```python
from build123d import *

# Parameters (mm, degrees)
SKETCH_1_W               = 120
SKETCH_1_H               = 80
EXTRUDE_1_DEPTH          = 5
SKETCH_3_R               = 4
CUT_EXTRUDE_2_DEPTH      = 10
SKETCH_5_R               = 15
CUT_EXTRUDE_3_DEPTH      = 10
F_4_0MM_1_D              = 4
FILLET_1_R               = 10
SKETCH_13_R              = 6.969385005
EXTRUDE_5_DEPTH          = 5
SKETCH_14_W              = 5
SKETCH_14_H              = 75
EXTRUDE_6_DEPTH          = 80
SKETCH_15_W              = 20
SKETCH_15_H              = 5
EXTRUDE_7_DEPTH          = 80
EXTRUDE_8_DEPTH          = 5
FILLET_2_R               = 1
F_3_0MM_1_D              = 3
F_3_0MM_1_DEPTH          = 7.5
F_3_0MM_1_TIP            = 0.901290929
SKETCH_21_R              = 2.5
CUT_EXTRUDE_7_DEPTH      = 10
PATTERN_CIRCULAR_1_COUNT = 4


with BuildPart() as part:
    # 草图1 → 凸台-拉伸1 (new body)
    with BuildSketch(Plane.XY):
        Rectangle(SKETCH_1_W, SKETCH_1_H)
    extrude(amount=EXTRUDE_1_DEPTH)

    # 草图3 → 切除-拉伸2 (cut)
    with BuildSketch(Plane.XY.offset(5)):
        with Locations((-45, 0)):
            Circle(SKETCH_3_R)
    extrude(amount=-CUT_EXTRUDE_2_DEPTH, mode=Mode.SUBTRACT)

    # 草图5 → 切除-拉伸3 (cut)
    with BuildSketch(Plane.XY.offset(5)):
        with Locations((35, 0)):
            Circle(SKETCH_5_R)
    extrude(amount=-CUT_EXTRUDE_3_DEPTH, mode=Mode.SUBTRACT)

    # Ø4.0mm 暗销孔1 (through all)
    with Locations(Plane(origin=(0, 0, 0), x_dir=(-1, 0, 0), z_dir=(0, 0, -1))):
        with Locations((-8.5, -22.25), (-8.5, 22.25), (-33.5, 22.25), (-33.5, -22.25)):
            Hole(F_4_0MM_1_D / 2)

    # 圆角1
    fillet_1_edges = [part.edges().sort_by_distance(p)[0] for p in [
        (-60, 40, 2.5),
        (-60, -40, 2.5),
    ]]
    fillet(fillet_1_edges, radius=FILLET_1_R)

    # 草图13 → 凸台-拉伸5 (add)
    with BuildSketch(Plane.XY.offset(5)):
        with Locations((-45, 0)):
            Circle(SKETCH_13_R)
    extrude(amount=-EXTRUDE_5_DEPTH)

    # 草图14 → 凸台-拉伸6 (add)
    with BuildSketch(Plane.XZ.offset(40)):
        with Locations((57.5, -37.5)):
            Rectangle(SKETCH_14_W, SKETCH_14_H)
    extrude(amount=-EXTRUDE_6_DEPTH)

    # 草图15 → 凸台-拉伸7 (add)
    with BuildSketch(Plane.XZ.offset(40)):
        with Locations((45, -72.5)):
            Rectangle(SKETCH_15_W, SKETCH_15_H)
    extrude(amount=-EXTRUDE_7_DEPTH)

    # 草图16 → 凸台-拉伸8 (add)
    with BuildSketch(Plane.XZ.offset(40)):
        Polygon((20, 5), (20, 0), (35, -55), (35, -75), (60, -75), (60, 5), align=None)
    extrude_8 = extrude(amount=-EXTRUDE_8_DEPTH)

    # 镜向1: 凸台-拉伸8 across plane
    add(extrude_8.mirror(Plane.ZX))

    # 圆角2
    fillet_2_edges = [part.edges().sort_by_distance(p)[0] for p in [
        (27.5, -40, -27.5),
        (-15, 40, 0),
        (60, 0, 5),
        (27.5, 40, -27.5),
        (5, 40, 5),
        (-15, -40, 0),
        (5, -40, 5),
        (-60, 0, 0),
        (-57.071067812, 37.071067812, 0),
        (-57.071067812, -37.071067812, 0),
        (-60, 0, 5),
        (-57.071067812, 37.071067812, 5),
        (-57.071067812, -37.071067812, 5),
        (60, 0, -75),
        (47.5, -40, -75),
        (47.5, 40, -75),
        (60, 40, -35),
        (60, -40, -35),
        (35, -40, -65),
        (35, 40, -65),
    ]]
    fillet(fillet_2_edges, radius=FILLET_2_R)

    # Ø3.0mm 暗销孔1
    with Locations(Plane.XY.offset(5)):
        with Locations((-5, -15), (-5, 15), (-20, 15), (-20, -15)):
            Hole(F_3_0MM_1_D / 2, depth=F_3_0MM_1_DEPTH)
            with Locations((0, 0, -(F_3_0MM_1_DEPTH + F_3_0MM_1_TIP / 2))):  # 118° drill point
                Cone(0, F_3_0MM_1_D / 2, F_3_0MM_1_TIP, mode=Mode.SUBTRACT)

    # 草图21 → 切除-拉伸7 (cut)
    with BuildSketch(Plane(origin=(60, 0, 0), x_dir=(0, 0, -1), z_dir=(1, 0, 0))):
        with Locations((35, 0)):
            Circle(SKETCH_21_R)
    extrude(amount=-CUT_EXTRUDE_7_DEPTH, mode=Mode.SUBTRACT)

    # 草图24 → Ø5.0mm 暗销孔1 (revolve, cut)
    with BuildSketch(Plane(origin=(60, 28.991378029, -6.008621971), x_dir=(0, 0, -1), z_dir=(0, 1, 0))):
        Polygon((0, 0), (0, 13.902151548), (2.5, 12.4), (2.5, 0), align=None)
    f_5_0mm_1 = revolve(axis=Axis((66.35, 28.991378029, -6.008621971), (-1, 0, 0)), mode=Mode.SUBTRACT)

    # 阵列(圆周)1: Ø5.0mm 暗销孔1 ×4 about axis
    pattern_circular_1_axis = Axis((0, 0, -35), (1, 0, 0))
    for i in range(1, PATTERN_CIRCULAR_1_COUNT):
        add(f_5_0mm_1.rotate(pattern_circular_1_axis, i * 360 / PATTERN_CIRCULAR_1_COUNT), mode=Mode.SUBTRACT)


solid = part.part
```
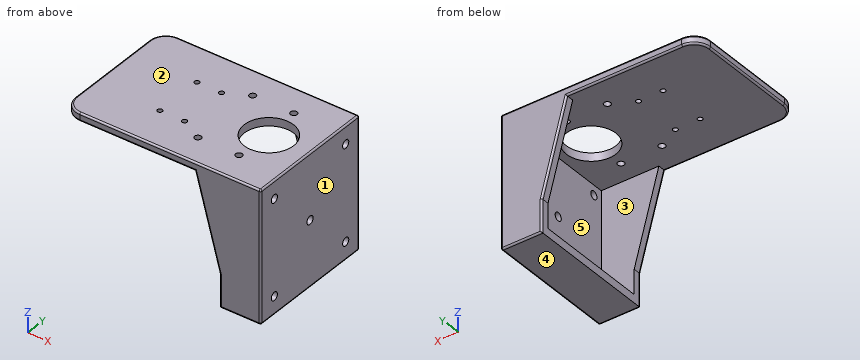
Can you work these out from the model? Positions are in its coordinate system, mm. Face numbers are marked on the shaded views. A direction names the side the tool comes from. Give positions to 0.01 mm unless a question says otherwise; leave off trailing zeros. Order: outer loops, then holes, each group sorted by start corner. A loop starts at its lowest first (then second) coordinate and runs counter-clockwise, first axis right, second up. Notation, with made-up numbers: (37.25, -40) - (89.25, -40) arc R8 cw to (89.25, -28) - close; hole circle Ø2 at (-24.5, 46.5). An arc over 180 degrees is marked (long way). Use a Markdown table: item, result. Add a question column.
Q1. If we mould it in two halves opening along Z, with no side actions, what happens to the marked faces 1, 2 and 3? For each: released by +Z, released by -Z, zero draft, split by the parting line, or undercut.
Q2. If we section it at B-B on y = 0: Write out the boundary of the cut face in (x, z).
Q3. If we section it at A-A on x = 8.5: Write out the boundary of the cut face in (y, z), plus the area to 3 significant figures.
Q4. On a 3-axis mill with a long thin cutter (end or side, diameter ignored), from which of +Z, -Z, +X, -X, +Y, -Y can I reach the whole of each face in a straight line? I mean the marked faces 4 and 5. Say none if no direction works.
Q5. Please list where these lines run through material, in increasing order: line 1 along Y through (x, z) = (-5, 3.45); line 2 along Y through (x, z) = (33.5, 3.35); line 3 along Y through (x, z) = (58, -35).
Q6. If we section it at D-D on y = -22.25: Write out the boundary of the cut face in (x, z).
Q7. I'm going to push flat-ended pins straight in: pin 1 (10 mm diameter, centred on x = -11, y = 9.5, fed in from -Z); pin 2 (4.5 mm diameter, centred on x = 33.5, y = -22.25, fed in from +Z); pin 3 (22 mm diameter, centred on y = -17, z = -68.5, fed in from -X); pin 4 (2 mm diameter, centred on y = 28.5, z = -38, fed in from -X). Where does each tip first touch, or does it pass through?
Q8. If we section it at C-C on x = -16: Write out the boundary of the cut face in (y, z).
Answers follow:
| question | item | result |
|---|---|---|
| 1 | face 1 | zero draft |
| 1 | face 2 | released by +Z |
| 1 | face 3 | undercut |
| 2 | outline | (-60, 1) arc R1 ccw to (-59, 0) - (20, 0) - (20, 5) - (-59, 5) arc R1 ccw to (-60, 4) - close; (35, -75) - (59, -75) arc R1 ccw to (60, -74) - (60, -37.5) - (55, -37.5) - (55, -70) - (35, -70) - close; (50, 0) - (55, 0) - (55, -32.5) - (60, -32.5) - (60, 4) arc R1 ccw to (59, 5) - (50, 5) - close |
| 3 | outline | (-40, 1) arc R1 ccw to (-39, 0) - (-24.25, 0) - (-24.25, 5) - (-39, 5) arc R1 ccw to (-40, 4) - close; (-20.25, 0) - (20.25, 0) - (20.25, 5) - (-20.25, 5) - close; (24.25, 0) - (39, 0) arc R1 ccw to (40, 1) - (40, 4) arc R1 ccw to (39, 5) - (24.25, 5) - close |
| 3 | area | 359 mm^2 |
| 4 | face 4 | -Z, +X, -X, +Y, -Y |
| 4 | face 5 | -X |
| 5 | line 1 | y = -40 to -16.5, -13.5 to 13.5, 16.5 to 40 |
| 5 | line 2 | y = -40 to -24.25, -20.25 to -14.92, 14.92 to 20.25, 24.25 to 40 |
| 5 | line 3 | y = -40 to -2.5, 2.5 to 40 |
| 6 | outline | (-60, 1) arc R1 ccw to (-59, 0) - (6.5, 0) - (6.5, 5) - (-59, 5) arc R1 ccw to (-60, 4) - close; (10.5, 0) - (31.5, 0) - (31.5, 5) - (10.5, 5) - close; (35, -75) - (59, -75) arc R1 ccw to (60, -74) - (60, 4) arc R1 ccw to (59, 5) - (35.5, 5) - (35.5, 0) - (55, 0) - (55, -70) - (35, -70) - close |
| 7 | pin 1 | stops at z = 0 |
| 7 | pin 2 | stops at z = 5 |
| 7 | pin 3 | stops at x = 35 |
| 7 | pin 4 | stops at x = 55 |
| 8 | outline | (-40, 1) arc R1 ccw to (-39, 0) - (39, 0) arc R1 ccw to (40, 1) - (40, 4) arc R1 ccw to (39, 5) - (-39, 5) arc R1 ccw to (-40, 4) - close |
